The model under review builds one solid part; all positions refer to its coordinate system, in mm. A direction names the side the tool comes from. Round coordinates to 2 decimals unless told otherwise and drop trailing zeros. Order: outer loops, then holes, each group sorted by start corner. A loop starts at its lowest first (then second) coordinate and runs counter-clockwise, first axis right, second up. Notation, with made-up numbers: (0.5, 62.25) - (25.5, 62.25) arc R33 cw to (25.5, 99.25) - close; hole circle Ø7 at (31.5, 26). An arc over 180 degrees is marked (long way). One line per question, with ' | ' between items. Start each with the question number.
Item 1: Draft analysis for pull direction Z (two halves, no side actions). For faces 5 (the face through (0, -56, 78)), 6 (the face through (3.698, -93.976, 40.678)), 7 (the face through (9, -2, -95)), 8 (the face through (9.37, -110.99, 58.04)), state which applies: +Z half, -Z half, draft (parallel to the pull), parting line (faces both ways), or undercut.
Item 2: Add section C-C on z = 43. State the section outline as (x, y) points, and give its area (3 significant figures).
Item 3: For L1, parallel to Y at x = 4, z = -61; L2, parallel to Z at x = 7, y = -3; L3, parallel to X at y = -83, z = 54.5, list the stretches that pass through material, from the lowest coordinate up. Write a range as [from, to].
Item 4: Add section A-A on x = 4.25. State the section outline as (y, z) points, and give its area (3 significant figures).
Item 5: Add section B-B on y = -12. State the section outline as (x, z) points.
Item 6: Tool access review of faces 1 (the face through (4, 64, 76)), 2 (the face through (3.698, -102.61, 46.015)), 3 (the face through (4, -131, -62)), 4 (the face through (9, -150, -62)): name each direction out of +Z, -Z, +X, -X, +Y, -Y from which nothing blocks a thin tool from reaching the whole face with its end or side.
Item 7: Insertion check: pin 1 Ø8 at (y, z) = (-53.5, 55.5) entering from -X. The pin has a flat end and moves straight along its axis. Give the tip position at first contact, or say it passes through.
from build123d import *

# Parameters (mm, degrees)
F1_DEPTH = 19
F3_DEPTH = 7.5


with BuildPart() as f1:
    # F0 (on Right) → F1 (new body)
    with BuildSketch(Plane.YZ):
        with BuildLine():
            Line((150, 95), (-25, 95))
            ThreePointArc((-25, 95), (-111.955644, 57.084235), (-150, -29.815225))
            Line((-150, -29.815225), (-150, -40))
            Line((-150, -40), (-150, -95))
            Line((-150, -95), (150, -95))
            Line((150, -95), (150, 95))
        make_face()
    extrude(amount=F1_DEPTH)

    # F2 (on face) → F3 (cut)
    with BuildSketch(Plane(origin=(0, 0, 0), x_dir=(0, -1, 0), z_dir=(-1, 0, 0))):
        with BuildLine():
            Line((25, 84), (-150, 84))
            Line((-150, 84), (-150, 76))
            Line((-150, 76), (25, 76))
            ThreePointArc((25, 76), (94.770081, 39.891752), (131, -29.815225))
            Line((131, -29.815225), (131, -95))
            Line((131, -95), (139, -95))
            Line((139, -95), (139, -29.815225))
            ThreePointArc((139, -29.815225), (101.75341, 46.877867), (25, 84))
        make_face()
    extrude(amount=-F3_DEPTH, mode=Mode.SUBTRACT)


solid = f1.part
Determined:
1) face 5: draft | face 6: undercut | face 7: -Z half | face 8: +Z half
2) outline: (0, -124.17) - (19, -124.17) - (19, 150) - (0, 150) - (0, -91.55) - (7.5, -91.55) - (7.5, -105.48) - (0, -105.48) - close | area: 5,100 mm2
3) L1: [-150, -139], [-131, 150] | L2: [-95, 76], [84, 95] | L3: [7.5, 19]
4) outline: (-150, -95) - (-139, -95) - (-139, -29.82) arc R130 cw to (-25, 84) - (150, 84) - (150, 95) - (-25, 95) arc R130 ccw to (-150, -29.82) - close; (-131, -95) - (150, -95) - (150, 76) - (-25, 76) arc R130 ccw to (-131, -29.82) - close | area: 49,900 mm2
5) outline: (0, -95) - (19, -95) - (19, 95) - (0, 95) - (0, 84) - (7.5, 84) - (7.5, 76) - (0, 76) - close
6) face 1: -X, +Y | face 2: -X | face 3: -Z, -X | face 4: +Z, -Z, +X, -X, -Y
7) pin 1: x = 0
